Autodesk Fusion 360 part; units mm, degrees
sketch "Sketch1" plane through (0, 0, 0) normal (0, 1, 0) x (1, 0, 0)
  line L0 (60, 0) -> (60, -30)
  line L1 (0, -15) -> (60, -15) construction
  line L2 (32, 0) -> (32, -30) construction
  line L3 (46, 0) -> (46, -30) construction
  line L4 (60, 0) -> (32, 0)
  line L5 (32, 0) -> (32, -30)
  line L6 (32, -30) -> (60, -30)
  line L7 (60, -30) -> (60, 0)
  dimension "d39" = 14
  dimension "d40" = 28
  dimension "d42" = 30
extrude "Extrude1" add sketch "Sketch1" along normal blind 9.6
sketch "Sketch2" plane through (0, 9.6, 0) normal (0, 1, 0) x (-1, 0, 0)
  line L0 (-60, 30) -> (-60, 0)
  circle A0 centre (-46, 15) radius 11.05
  circle A1 centre (-46, 15) radius 10.55
  line L1 (-60, 0) -> (-32, 0)
  line L2 (-32, 0) -> (-32, 30)
  line L3 (-32, 30) -> (-60, 30)
  dimension "d15" = 22.1
  dimension "d16" = 21.1
extrude "Extrude2" cut sketch "Sketch2" against normal blind 7 contours A0
extrude "Extrude3" cut 1 faces at (43.0944, 9.6, 14.0673) along direction (0, 1, 0) through all and the other way through all
sketch "Sketch3" plane through (0, 9.6, 0) normal (0, 1, 0) x (-1, 0, 0)
  line L0 (-60, 30) -> (-60, 0)
  circle A0 centre (-46, 15) radius 13 construction
  line L1 (-32, 30) -> (-60, 30)
  line L2 (-60, 0) -> (-32, 0)
  line L3 (-32, 0) -> (-32, 30)
  circle A1 centre (-46, 15) radius 11.05
  point P0 (-35.8444, 6.8844)
  point P1 (-55.1828, 24.202)
  point P2 (-56.1556, 6.8844)
  dimension "d30" = 26
hole "Hole1" at (35.8444, 9.6, 6.8844) direction (0, -1, 0) diameter 2.5 end through all
hole "Hole2" at (56.1556, 9.6, 6.8844) direction (0, -1, 0) diameter 2.5 end through all
hole "Hole3" at (55.1828, 9.6, 24.202) direction (0, -1, 0) diameter 2.5 end through all
sketch "Sketch4" plane through (0, 0, 0) normal (0, 0, -1) x (-1, 0, 0)
  line L0 (-60, 0) -> (-32, 0)
  line L1 (-32, 0) -> (-32, 9.6)
  line L2 (-32, 9.6) -> (-60, 9.6)
  line L3 (-60, 9.6) -> (-60, 0)
  line L4 (-32, 4.8) -> (-60, 4.8) construction
  line L5 (-39, 0) -> (-39, 9.6) construction
  line L6 (-53, 0) -> (-53, 9.6) construction
  point P0 (-39, 4.8)
  point P1 (-53, 4.8)
  dimension "d43" = 14
  dimension "d44" = 7
hole "Hole4" at (39, 4.8, 0) direction (0, 0, 1) diameter 3.3 depth 4 tip angle 118
hole "Hole5" at (53, 4.8, 0) direction (0, 0, 1) diameter 3.3 depth 4 tip angle 118
Design review of the part built by this model. Coordinates are the model's own, in mm. A direction names the side the tool comes from. Coordinates: 2 decimals unless noted, no trailing zeros. Order: outer loops, then holes, each group sorted by start corner. A loop starts at its lowest first (then second) coordinate and runs counter-clockwise, first axis right, second up.
Item 1: For faces 5 (the cylindrical face through (51.61, 5.69, 2.03)), 6 (the flat face through (46, 5, 0)), 7 (the flat face through (42, 2.6, 5)), list the 3-axis set-ups (+Z, -Z, +X, -X, +Y, -Y) from which the entire face can be reached by the end or side of a thin tool; tool diameter is ignored.
Item 2: For line 1 (X direction, y = 4.8, z = 2.35); line 2 (Y direction, x = 53, z = 2.8); line 3 (X direction, y = 1.5, z = 13.25), list the stretches that pass through material, from the lowest coordinate up.
Item 3: Take a section at B-B, the plane x = 46. Write out the cut boundary in (y, z).
Item 4: The part is to be moulded in two halves that separate along X. For faces 1 (the flat face through (60, 5, 15)), 2 (the flat face through (46, 5, 30)), 3 (the flat face through (32, 5, 15)), 4 (the cylindrical face through (34.605, 4.733, 6.722)), say which applies: pulls with the +X half, pulls with the -X half, needs draft (parallel to the pull), parting line crosses it, or undercut.
Item 5: Take a section at C-C, the plane z = 7.5. Write out the cut boundary in (x, y), then the cut area to 3 significant figures.
Item 6: Take a section at D-D, the plane y = 9.25. Write out the cut boundary in (x, z).
Item 7: For pin 1 Ø1 at (x, z) = (40.5, 4) entering from -Y; pin 2 Ø2.5 at (x, y) = (53, 4.8) entering from -Z, all flat-tipped, find the tip position at first contact; note any pin that passes through.
Item 8: Take a section at A-A, the plane z = 15. Write out the cut boundary in (x, y), then the cut area to 3 significant figures.
The answers:
1. face 5: -Z
1. face 6: -Z, +X, -X, +Y, -Y
1. face 7: +Y
2. line 1: x = 32 to 37.35, 40.65 to 51.35, 54.65 to 60
2. line 2: y = 0 to 3.15, 6.45 to 9.6
2. line 3: x = 32 to 35.6, 56.4 to 60
3. outline: (0, 0) - (9.6, 0) - (9.6, 3.95) - (2.6, 3.95) - (2.6, 4.45) - (0, 4.45) - close; (0, 25.55) - (2.6, 25.55) - (2.6, 26.05) - (9.6, 26.05) - (9.6, 30) - (0, 30) - close
4. face 1: pulls with the +X half
4. face 2: needs draft
4. face 3: pulls with the -X half
4. face 4: undercut
5. outline: (32, 0) - (34.76, 0) - (34.76, 9.6) - (32, 9.6) - close; (36.93, 0) - (38.58, 0) - (38.58, 2.6) - (37.89, 2.6) - (37.89, 9.6) - (36.93, 9.6) - close; (53.42, 0) - (55.07, 0) - (55.07, 9.6) - (54.11, 9.6) - (54.11, 2.6) - (53.42, 2.6) - close; (57.24, 0) - (60, 0) - (60, 9.6) - (57.24, 9.6) - close
5. area: 74.8 mm2
6. outline: (32, 0) - (60, 0) - (60, 30) - (32, 30) - close; hole circle Ø2.5 at (35.84, 6.88); hole circle Ø22.1 at (46, 15); hole circle Ø2.5 at (55.18, 24.2); hole circle Ø2.5 at (56.16, 6.88)
7. pin 1: stops at y = 0
7. pin 2: stops at z = 4.24
8. outline: (32, 0) - (35.45, 0) - (35.45, 2.6) - (34.95, 2.6) - (34.95, 9.6) - (32, 9.6) - close; (56.55, 0) - (60, 0) - (60, 9.6) - (57.05, 9.6) - (57.05, 2.6) - (56.55, 2.6) - close
8. area: 59.2 mm2
